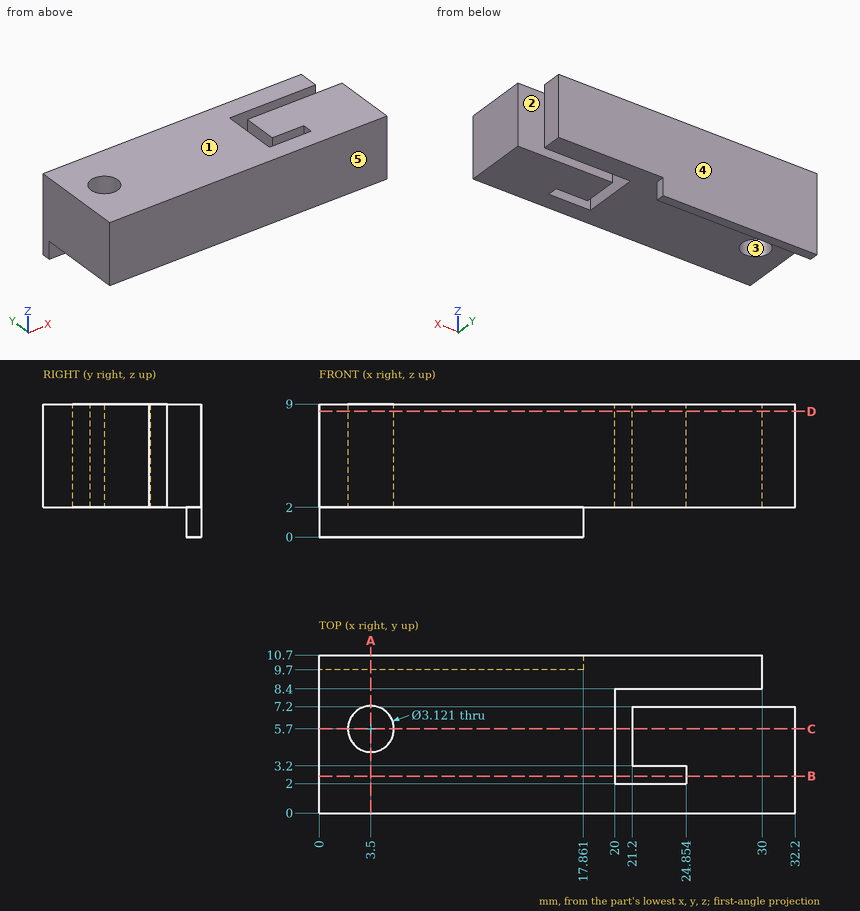
Verification items for this drawing (mm, ordinates from the low corner). A direction names the side the tool comes from. Coordinates: 2 decimals unless noted, no trailing zeros. Write each loop counter-clockwise with the first axis right and the second up, starting at its lowest first coordinate (ties: lowest second). Pieces come first, ordered by that corner, then holes. Notation, with made-up numbers: M 42,65.5 L 70,65.5 A10 cw 70,77.5 Z; hole C -15.75,-10 d8. An arc over 180 degrees is marked long. Use one line per item in the form item = value. Start each with the question number.
1) Go/stop test with flat-tipped pins: pin 1 Ø0.7 at (y, z) = (9.5, 4) entering from +X; pin 2 Ø3 at (x, y) = (19.5, 8.5) entering from -Z; pin 3 Ø1 at (x, z) = (7.5, 0.5) entering from -Y. Record where each tip stops, or that it passes through.
2) Section check D-D on z = 8.5. Enter the section's corners in (x, y).
3) Release check for a two-part mould opening along Y. For the marked faces 3, 4 and 5 record: pulls with the +Y half, pulls with the -Y half, needs draft (parallel to the pull), parting line crosses it, or undercut.
4) Thickness scan on probe 1 along Y at (x, z) = (21, 5.5); probe 2 along X at (y, z) = (4, 4.75); probe 3 along Y at (x, z) = (3.5, 4.25). Record the ranges inside material, lowest first. Write a range as from..to.
5) Section check C-C on y = 5.7. Enter the section's corners in (x, z), and give its area (3 significant figures).
6) Section check B-B on y = 2.5. Enter the section's corners in (x, z).
7) Set-up check for the marked faces 1 and 2: record each of +Z, -Z, +X, -X, +Y, -Y from which the full face is reachable in a straight line by a thin tool's end or side.
8) Section check A-A on x = 3.5. Enter the section's corners in (y, z).
Responses:
q1.pin_1 = 30
q1.pin_2 = 2
q1.pin_3 = 9.7
q2.outline = M 0,0 L 32.2,0 L 32.2,7.2 L 21.2,7.2 L 21.2,3.2 L 24.85,3.2 L 24.85,2 L 20,2 L 20,8.4 L 30,8.4 L 30,10.7 L 0,10.7 Z; hole C 3.5,5.7 d3.12
q3.face_3 = undercut
q3.face_4 = pulls with the +Y half
q3.face_5 = pulls with the -Y half
q4.probe_1 = 0..2, 8.4..10.7
q4.probe_2 = 0..20, 21.2..32.2
q4.probe_3 = 0..4.14, 7.26..10.7
q5.outline = M 0,2 L 1.94,2 L 1.94,9 L 0,9 Z; M 5.06,2 L 20,2 L 20,9 L 5.06,9 Z; M 21.2,2 L 32.2,2 L 32.2,9 L 21.2,9 Z
q5.area = 195 mm2
q6.outline = M 0,2 L 20,2 L 20,9 L 0,9 Z; M 24.85,2 L 32.2,2 L 32.2,9 L 24.85,9 Z
q7.face_1 = +Z, +X, -X, +Y, -Y
q7.face_2 = +Z, -Z, +X
q8.outline = M 0,2 L 4.14,2 L 4.14,9 L 0,9 Z; M 7.26,2 L 9.7,2 L 9.7,0 L 10.7,0 L 10.7,9 L 7.26,9 Z
